Verification items for the finished model (mm, model axes). Coordinates: 2 decimals unless noted, no trailing zeros. Loops run counter-clockwise (first coordinate to the right, second up) from the corner with the lowest first, then second, coordinate; pieces in that order, holes last. Notation, with made-up numbers: (44, -32) -> (88, -32) arc R25 cw to (88, -12) -> close; hole circle Ø6 at (62, 84.25). An arc over 180 degrees is marked (long way). Write item = value, one per line.
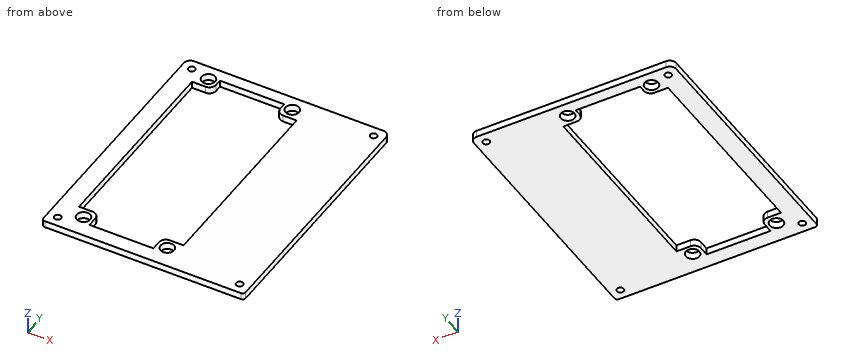
```python
from build123d import *

# Parameters (mm, degrees)
SKETCH_2_R          = 1
EXTRUDE_1_DEPTH     = 2
SKETCH_4_R          = 2
CUT_EXTRUDE_1_DEPTH = 3


with BuildPart() as part:
    # 草图2 → 凸台-拉伸1 (new body)
    with BuildSketch(Plane.XY):
        with BuildLine():
            Line((-56.473572366, -0.89607242), (1.526427634, -0.89607242))
            ThreePointArc((1.526427634, -0.89607242), (2.162823737, -0.632468523), (2.426427634, 0.00392758))
            Line((2.426427634, 0.00392758), (2.426427634, 72.00392758))
            ThreePointArc((2.426427634, 72.00392758), (1.869930519, 73.347430464), (0.526427634, 73.90392758))
            Line((0.526427634, 73.90392758), (-55.473572366, 73.90392758))
            ThreePointArc((-55.473572366, 73.90392758), (-56.81707525, 73.347430464), (-57.373572366, 72.00392758))
            Line((-57.373572366, 72.00392758), (-57.373572366, 0.00392758))
            ThreePointArc((-57.373572366, 0.00392758), (-57.109968469, -0.632468523), (-56.473572366, -0.89607242))
        make_face()
        with Locations((-54.373572366, 70.90392758)):
            Circle(SKETCH_2_R, mode=Mode.SUBTRACT)
        with Locations((-0.573572366, 70.90392758)):
            Circle(SKETCH_2_R, mode=Mode.SUBTRACT)
        with Locations((-0.573572366, 2.10392758)):
            Circle(SKETCH_2_R, mode=Mode.SUBTRACT)
        with Locations((-54.373572366, 2.10392758)):
            Circle(SKETCH_2_R, mode=Mode.SUBTRACT)
    extrude(amount=EXTRUDE_1_DEPTH)

    # 草图4 → 切除-拉伸1 (cut)
    with BuildSketch(Plane.XY):
        with BuildLine():
            Line((-51.773572366, 66.50392758), (-51.773572366, 8.50392758))
            Line((-51.773572366, 8.50392758), (-47.786382689, 8.50392758))
            ThreePointArc((-47.786382689, 8.50392758), (-46.372169126, 7.918141142), (-45.786382689, 6.50392758))
            Line((-45.786382689, 6.50392758), (-45.786382689, 3.50392758))
            Line((-45.786382689, 3.50392758), (-26.886382689, 3.50392758))
            Line((-26.886382689, 3.50392758), (-26.886382689, 6.40392758))
            ThreePointArc((-26.886382689, 6.40392758), (-26.300596251, 7.818141142), (-24.886382689, 8.40392758))
            Line((-24.886382689, 8.40392758), (-20.773572366, 8.40392758))
            Line((-20.773572366, 8.40392758), (-20.773572366, 66.40392758))
            Line((-20.773572366, 66.40392758), (-24.773572366, 66.40392758))
            ThreePointArc((-24.773572366, 66.40392758), (-26.187785928, 66.989714017), (-26.773572366, 68.40392758))
            Line((-26.773572366, 68.40392758), (-26.773572366, 70.45392758))
            Line((-26.773572366, 70.45392758), (-45.786382689, 70.45392758))
            Line((-45.786382689, 70.45392758), (-45.786382689, 68.50392758))
            ThreePointArc((-45.786382689, 68.50392758), (-46.372169126, 67.089714017), (-47.786382689, 66.50392758))
            Line((-47.786382689, 66.50392758), (-51.773572366, 66.50392758))
        make_face()
        with Locations(Location((-23.873572366, 69.55392758, 0), (0, 0, 180))):
            Circle(SKETCH_4_R)
        with Locations(Location((-48.673572366, 69.55392758, 0), (0, 0, 180))):
            Circle(SKETCH_4_R)
        with Locations(Location((-48.673572366, 5.45392758, 0), (0, 0, 180))):
            Circle(SKETCH_4_R)
        with Locations(Location((-23.873572366, 5.45392758, 0), (0, 0, 180))):
            Circle(SKETCH_4_R)
    extrude(amount=CUT_EXTRUDE_1_DEPTH, mode=Mode.SUBTRACT)


solid = part.part
```
1) Sectioned sample at A-A, the plane y = 22.5. Record the cut outline in (x, z), plus the area to 3 significant figures.
Ans:
outline = (-57.37, 0) -> (-51.77, 0) -> (-51.77, 2) -> (-57.37, 2) -> close; (-20.77, 0) -> (2.43, 0) -> (2.43, 2) -> (-20.77, 2) -> close
area = 57.6 mm2
2) Sectioned sample at B-B, the plane x = -40. Record the cut outline in (y, z), plus the area to 3 significant figures.
Ans:
outline = (-0.9, 0) -> (3.5, 0) -> (3.5, 2) -> (-0.9, 2) -> close; (70.45, 0) -> (73.9, 0) -> (73.9, 2) -> (70.45, 2) -> close
area = 15.7 mm2
3) Sectioned sample at C-C, the plane z = 1.4. Count the separate pieces of the cut face and the enclosed holes in it, plus the area to 3 significant figures.
Ans:
separate_pieces = 1
enclosed_holes = 9
area = 2,440 mm2
4) Material ranges on line 1 (X direction, y = 17, z = 1.2); line 2 (Y direction, x = -51.5, z = 0.85); line 3 (Y direction, x = -24, z = 0.7), recorded low to high.
Ans:
line_1 = -57.37 to -51.77, -20.77 to 2.43
line_2 = -0.9 to 8.5, 66.5 to 73.9
line_3 = -0.9 to 3.46, 7.45 to 8.4, 66.4 to 67.56, 71.55 to 73.9
5) Sectioned sample at D-D, the plane x = -23. Record the cut outline in (y, z), plus the area to 3 significant figures.
Ans:
outline = (-0.9, 0) -> (3.65, 0) -> (3.65, 2) -> (-0.9, 2) -> close; (7.25, 0) -> (8.4, 0) -> (8.4, 2) -> (7.25, 2) -> close; (66.4, 0) -> (67.75, 0) -> (67.75, 2) -> (66.4, 2) -> close; (71.35, 0) -> (73.9, 0) -> (73.9, 2) -> (71.35, 2) -> close
area = 19.2 mm2
